from build123d import *

# Parameters (mm, degrees)
SWEEP1_PROFILE_R   = 37.5
SHELL1_T           = -10
CUT_EXTRUDE1_REACH = 264.797
SKETCH4_R          = 27.5


with BuildPart() as part:
    # Sweep1: sweep along a path in Sketch2
    with BuildLine(Plane(origin=(0, 0, 0), x_dir=(1, 0, 0), z_dir=(0, 1, 0))) as sweep1_path:
        Line((150, 0), (0, 0))
        ThreePointArc((0, 0), (-53.033008589, 21.966991411), (-75, 75))
        Line((-75, 75), (-75, 175))
    # Sweep1 profile (on start of the path) → Sweep1 (sweep)
    with BuildSketch(Plane(origin=(150, 0, 0), x_dir=(0, 0, -1), z_dir=(-1, 0, 0))):
        Circle(SWEEP1_PROFILE_R)
    sweep(path=sweep1_path.line)

    # Shell1
    shell1_openings = [part.faces().sort_by_distance(p)[0] for p in [
        (150, 0, 0),
    ]]
    offset(amount=SHELL1_T, openings=shell1_openings, kind=Kind.INTERSECTION)

    # Sketch4 → Cut-Extrude1 (cut, up to next)
    with BuildSketch(Plane(origin=(0, 0, -175), x_dir=(-1, 0, 0), z_dir=(0, 0, -1)), mode=Mode.PRIVATE) as cut_extrude1_sk1:
        with Locations((75, 0)):
            Circle(SKETCH4_R)
    cut_extrude1_tool1 = extrude(cut_extrude1_sk1.sketch, amount=-CUT_EXTRUDE1_REACH, mode=Mode.PRIVATE) & part.part
    add(cut_extrude1_tool1.solids().sort_by_distance((-75, 0, -175))[0], mode=Mode.SUBTRACT)


solid = part.part
CAD build for the part. Positions are in the model's coordinates, mm. A direction names the side the tool comes from. Give positions to 0.01 mm unless a question says otherwise; leave off trailing zeros. Loops run counter-clockwise (first coordinate to the right, second up) from the corner with the lowest first, then second, coordinate; pieces in that order, holes last. Notation, with made-up numbers: M 73,-26.5 L 120,-26.5 A27 cw 120,-9.5 Z; hole C 54.5,16 d8. An arc over 180 degrees is marked long. One line per question, with ' | ' between items. Start each with the question number.
1. Two-plate mould, pull along Z, no slides. Class faces 3 (the face through (-55, 20, -175)), 4 (the face through (150, -20, 20)), 5 (the face through (73.95, 26.846, 5.961)): pulls with the +Z half, pulls with the -Z half, needs draft (parallel to the pull), parting line crosses it, or undercut.
2. Flat gauge pins, fed straight in: pin 1 (8 mm diameter, centred on y = 4.5, z = -41, fed in from -X); pin 2 (10 mm diameter, centred on x = -45, y = 28.5, fed in from +Z); pin 3 (1.5 mm diameter, centred on x = 40, y = -3.5, fed in from -Z). Where does each tip first touch, or does it go through?
3. Saw through at A-A on y = 0. Give the cut face in (x, z).
4. 3-axis set-ups, long thin cutter, end or side, ignore diameter. For faces 1 (the face through (73.95, -37.18, 4.88)), 2 (the face through (-39.23, -11.26, -125.7)): which of +Z, -Z, +X, -X, +Y, -Y reach the whole face in a straight line?
5. Probe L1, parallel to Z at x = 44.5, y = 0; L2, parallel to X at y = 0, z = -172.25. List the from-to ranges inside material, lowest first. Write a range as from..to.
6. Saw through at B-B on x = 82. Give the cut face in (y, z), plus the area to 3 significant figures.
7. Saw through at C-C on z = -156. Give the cut face in (x, y).
8. Saw through at D-D on y = 24.5. Give the cut face in (x, z), plus the area to 3 significant figures.
Result sheet:
1) face 3: pulls with the -Z half | face 4: needs draft | face 5: undercut
2) pin 1: stops at x = -108.22 | pin 2: stops at z = 19.57 | pin 3: stops at z = -37.4
3) outline: M -112.5,-175 L -102.5,-175 L -102.5,-75 A102.5 cw 0,27.5 L 150,27.5 L 150,37.5 L 0,37.5 A112.5 ccw -112.5,-75 Z; M -47.5,-175 L -37.5,-175 L -37.5,-75 A37.5 cw 0,-37.5 L 150,-37.5 L 150,-27.5 L 0,-27.5 A47.5 ccw -47.5,-75 Z
4) face 1: +X | face 2: -Z
5) L1: z = -37.5..-27.5, 27.5..37.5 | L2: x = -112.5..-102.5, -47.5..-37.5
6) outline: C 0,0 d75; hole C 0,0 d55 | area: 2,040 mm^2
7) outline: C -75,0 d75; hole C -75,0 d55
8) outline: M -103.39,-175 L -87.49,-175 L -87.49,-75 A87.49 cw 0,12.49 L 150,12.49 L 150,28.39 L 0,28.39 A103.39 ccw -103.39,-75 Z; M -62.51,-175 L -46.61,-175 L -46.61,-75 A46.61 cw 0,-28.39 L 150,-28.39 L 150,-12.49 L 0,-12.49 A62.51 ccw -62.51,-75 Z | area: 11,700 mm^2
